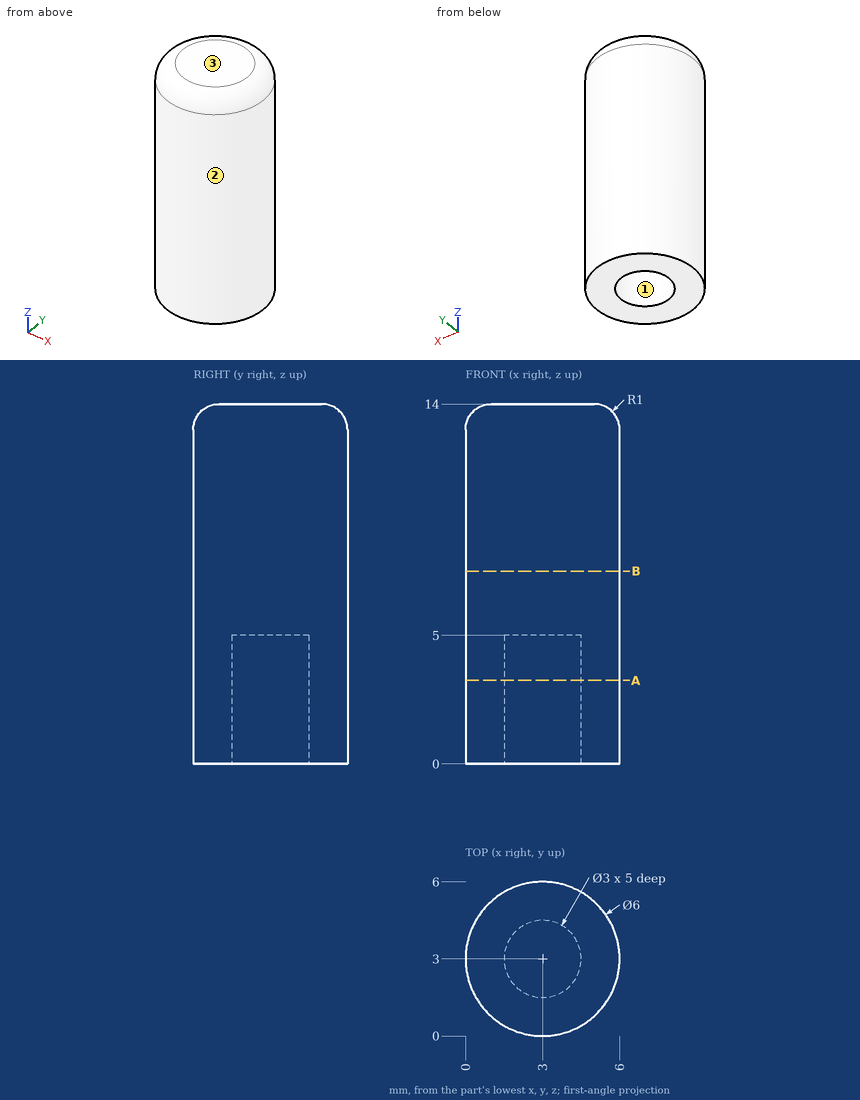
Print and shaded views of the part. All mm, measured from the part's lowest x, y and z. Round coordinates to 2 decimals unless told otherwise and drop trailing zeros. Loops run counter-clockwise (first coordinate to the right, second up) from the corner with the lowest first, then second, coordinate; pieces in that order, holes last. Notation, with made-up numbers: (12.5, 38) -> (64.5, 38) arc R23 cw to (64.5, 61) -> close; hole circle Ø8 at (84.5, 9.5). An arc over 180 degrees is marked (long way). Use CSV: the item, a comma, the result in double quotes. Start each with the question number.
1) Drop a flat-ended pin along its axis: P1, Ø1.5, axis at x = 1, z = 5.5, coming from the -Y side. Give the stop position or say it passes through.
2) Cut at A-A, the plane z = 3.25. Write the cut outline in (x, y), plus the area to 3 significant figures.
3) Pull direction Y, two halves, no side cores. Call the marked faces 1, 2 and 3: +Y half, -Y half, draft (parallel to the pull), parting line (faces both ways), or undercut.
4) Wall check: L1, parallel to Y at x = 3, z = 1.55; L2, parallel to Z at x = 3.25, y = 2.25; L3, parallel to Y at x = 4, z = 0.5. Give the ranges that are in metal, low to high. Write a range as [from, to].
5) Cut at B-B, the plane z = 7.5. Write the cut outline in (x, y), plus the area to 3 significant figures.
Determined:
1,P1,"stops at y = 0.27"
2,outline,"circle Ø6 at (3, 3); hole circle Ø3 at (3, 3)"
2,area,"21.2 mm2"
3,face 1,"undercut"
3,face 2,"parting line"
3,face 3,"draft"
4,L1,"y = [0, 1.5], [4.5, 6]"
4,L2,"z = [5, 14]"
4,L3,"y = [0.17, 1.88], [4.12, 5.83]"
5,outline,"circle Ø6 at (3, 3)"
5,area,"28.3 mm2"
